Could you check a few things on this model? Use its own coordinates, in mm. Give positions to 0.01 mm unless a question says otherwise; leave off trailing zeros. Order: outer loops, then holes, each group sorted by start corner. A loop starts at its lowest first (then second) coordinate and runs counter-clockwise, first axis right, second up.
from build123d import *

# Parameters (mm, degrees)
BOSS_EXTRUDE1_DEPTH      = 1.5875
BOSS_EXTRUDE1_DEPTH_BACK = 1.5875
SKETCH1_W                = 75
SKETCH1_H                = 60
CUT_EXTRUDE1_DEPTH       = 49.049663435
CUT_EXTRUDE1_DEPTH_BACK  = 49.049663435
SKETCH2_R                = 2.6


with BuildPart() as part:
    # Sketch1 → Boss-Extrude1 (new, two sides: drawn at the far end of the back side and taken through both)
    with BuildSketch(Plane(origin=(0, 0, 0), x_dir=(0, 0, -1), z_dir=(1, 0, 0)).offset(-BOSS_EXTRUDE1_DEPTH_BACK)):
        Rectangle(SKETCH1_W, SKETCH1_H)
    extrude(amount=BOSS_EXTRUDE1_DEPTH + BOSS_EXTRUDE1_DEPTH_BACK)

    # Sketch2 → Cut-Extrude1 (cut, two sides: drawn at the far end of the back side and taken through both)
    with BuildSketch(Plane(origin=(0, 0, 0), x_dir=(0, 0, -1), z_dir=(1, 0, 0)).offset(-CUT_EXTRUDE1_DEPTH_BACK)):
        with Locations((-31.05, 23.55)):
            Circle(SKETCH2_R)
        with Locations(Location((31.05, 23.55, 0), (0, 0, 180))):
            Circle(SKETCH2_R)
        with Locations((31.05, -23.55)):
            Circle(SKETCH2_R)
        with Locations(Location((-31.05, -23.55, 0), (0, 0, 180))):
            Circle(SKETCH2_R)
    extrude(amount=CUT_EXTRUDE1_DEPTH + CUT_EXTRUDE1_DEPTH_BACK, mode=Mode.SUBTRACT)


solid = part.part
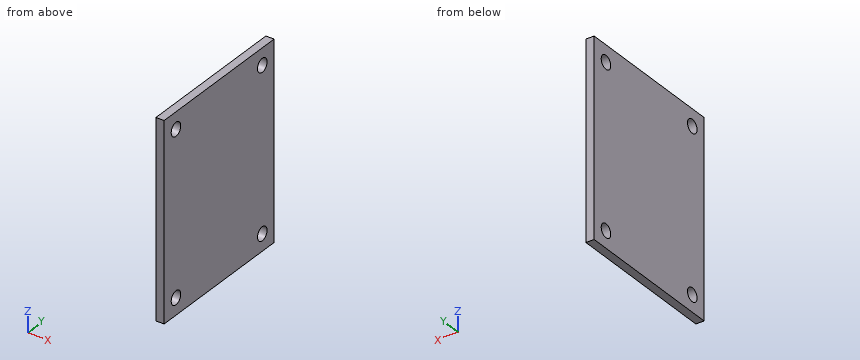
Item 1: Please list where these lines run through material, in increasing order: line 1 along Y through (x, z) = (0.8, 31.05); line 2 along Y through (x, z) = (-1.1, 33); line 3 along Z through (x, y) = (-0.8, -24).
Findings:
line 1: y = -30 to -26.15, -20.95 to 20.95, 26.15 to 30
line 2: y = -30 to -25.27, -21.83 to 21.83, 25.27 to 30
line 3: z = -37.5 to -33.61, -28.49 to 28.49, 33.61 to 37.5
Item 2: Imagine slicing it at A-A on y = 23.55. List the corners of the cut face in (x, z) for me, then the cut area to 3 significant figures.
Findings:
outline: (-1.59, -37.5) - (1.59, -37.5) - (1.59, -33.65) - (-1.59, -33.65) - close; (-1.59, -28.45) - (1.59, -28.45) - (1.59, 28.45) - (-1.59, 28.45) - close; (-1.59, 33.65) - (1.59, 33.65) - (1.59, 37.5) - (-1.59, 37.5) - close
area: 205 mm2
Item 3: Imagine slicing it at C-C on x = -1. List the corners of the cut face in (y, z) for me, then the cut area to 3 significant figures.
Findings:
outline: (-30, -37.5) - (30, -37.5) - (30, 37.5) - (-30, 37.5) - close; hole circle Ø5.2 at (-23.55, -31.05); hole circle Ø5.2 at (-23.55, 31.05); hole circle Ø5.2 at (23.55, -31.05); hole circle Ø5.2 at (23.55, 31.05)
area: 4,420 mm2
Item 4: Imagine slicing it at B-B on z = -31.05. List the corners of the cut face in (x, y) for me, then the cut area to 3 significant figures.
Findings:
outline: (-1.59, -30) - (1.59, -30) - (1.59, -26.15) - (-1.59, -26.15) - close; (-1.59, -20.95) - (1.59, -20.95) - (1.59, 20.95) - (-1.59, 20.95) - close; (-1.59, 26.15) - (1.59, 26.15) - (1.59, 30) - (-1.59, 30) - close
area: 157 mm2
